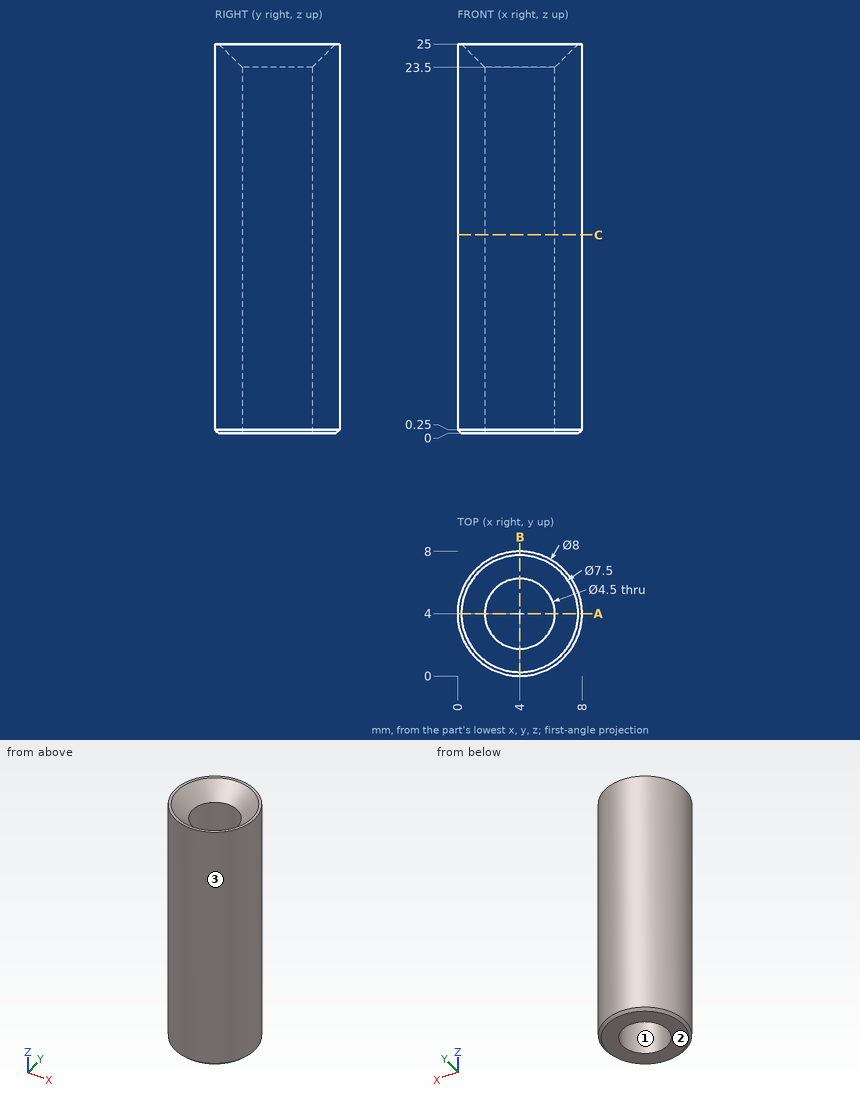
Can you work these out from the drawing? Everything is in mm from the part's minimum corner. Give positions to 0.01 mm unless a question says otherwise; leave off trailing zeros. Loops run counter-clockwise (first coordinate to the right, second up) from the corner with the lowest first, then second, coordinate; pieces in that order, holes last. Notation, with made-up numbers: (32, 39.25) -> (62, 39.25) arc R28 ccw to (62, 72.25) -> close; hole circle Ø1 at (13, 5.5). An arc over 180 degrees is marked (long way). Return JSON: item names as keys, results as strings.
Item 1: If we section it at A-A on y = 4: List the corners of the cut face in (x, z) for me.
Geometry results:
{"outline": "(0, 0.25) -> (0.25, 0) -> (1.75, 0) -> (1.75, 23.5) -> (0.25, 25) -> (0, 25) -> close; (6.25, 0) -> (7.75, 0) -> (8, 0.25) -> (8, 25) -> (7.75, 25) -> (6.25, 23.5) -> close"}
Item 2: If we section it at C-C on z = 12.75: List the corners of the cut face in (x, y) for me, plus the area to 3 significant figures.
Geometry results:
{"outline": "circle Ø8 at (4, 4); hole circle Ø4.5 at (4, 4)", "area": "34.4 mm²"}
Item 3: I need wall thicknesses on L1, parallel to Y at x = 4, z = 9.25; L2, parallel to X at y = 6, z = 20.25; L3, parallel to Y at x = 4.75, z = 6. Which ranges of each line are inside material? Lowest first, please. Write a range as from..to.
Geometry results:
{"L1": "y = 0..1.75, 6.25..8", "L2": "x = 0.54..2.97, 5.03..7.46", "L3": "y = 0.07..1.88, 6.12..7.93"}
Item 4: I'm going to push flat-ended pins straight in: pin 1 (1 mm diameter, centred on x = 5.5, y = 5.5, fed in from +Z); pin 2 (1.5 mm diameter, centred on x = 6.5, z = 16.5, fed in from -Y). Where does each tip first touch, or does it pass through?
Geometry results:
{"pin 1": "stops at z = 23.87", "pin 2": "stops at y = 0.4"}
Item 5: We'd pull the mould along X, two halves only. Please class the marked faces 1, 2 and 3: +X half, -X half, draft (parallel to the pull), parting line (faces both ways), or undercut.
Geometry results:
{"face 1": "undercut", "face 2": "draft", "face 3": "parting line"}
